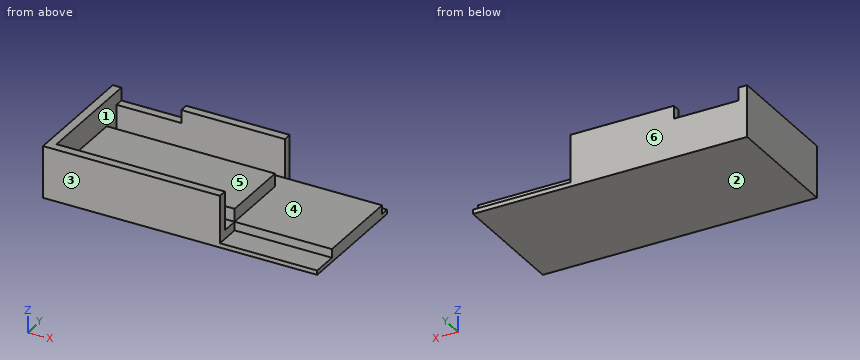
```python
from build123d import *

# Parameters (mm, degrees)
F0_W     = 39
F0_H     = 4
F0_W_2   = 2.54
F0_H_2   = 20.5
F1_DEPTH = 3
F0_H_3   = 16.5
F2_DEPTH = 6
F0_W_3   = 15
F0_H_4   = 2
F3_DEPTH = 9
F0_W_4   = 24
F4_DEPTH = 12
F5_DEPTH = 1


with BuildPart() as f1:
    # F0 (on Top) → F1 (new body)
    with BuildSketch(Plane.XY):
        Polygon((61, 26.5), (41, 26.5), (41, 22.5), (41, 6), (61, 6), align=None)
        Polygon((17, 26.5), (2, 26.5), (2, 22.5), (41, 22.5), (41, 26.5), align=None)
        with Locations((21.5, 4)):
            Rectangle(F0_W, F0_H)
        with Locations((62.27, 16.25)):
            Rectangle(F0_W_2, F0_H_2)
    extrude(amount=F1_DEPTH)

    # F0 (on Top) → F3 (join)
    with BuildSketch(Plane.XY):
        with Locations((9.5, 27.5)):
            Rectangle(F0_W_3, F0_H_4)
    extrude(amount=F3_DEPTH)



with BuildPart() as f2:
    # F0 (on Top) → F2 (new body)
    with BuildSketch(Plane.XY):
        with Locations((21.5, 14.25)):
            Rectangle(F0_W, F0_H_3)
    extrude(amount=F2_DEPTH)


with BuildPart() as f4:
    # F0 (on Top) → F4 (new body)
    with BuildSketch(Plane.XY):
        with Locations((29, 27.5)):
            Rectangle(F0_W_4, F0_H_4)
        Polygon((2, 22.5), (2, 26.5), (2, 28.5), (0, 28.5), (0, 2), (2, 2), (2, 6), align=None)
        Polygon((41, 2), (2, 2), (0, 2), (0, 0), (41, 0), align=None)
    extrude(amount=F4_DEPTH)


with BuildPart() as f1_1:
    add(f1.part)

    add(f2.part)  # F5 merges F2

    add(f4.part)  # F5 merges F4
    # F0 (on Top) → F5 (join)
    with BuildSketch(Plane.XY):
        Polygon((41, 28.5), (41, 26.5), (61, 26.5), (63.54, 26.5), (63.54, 28.5), align=None)
        Polygon((61, 6), (41, 6), (41, 2), (41, 0), (63.54, 0), (63.54, 6), align=None)
    extrude(amount=F5_DEPTH)


solid = f1_1.part
```
Could you check a few things on this model? Use its own coordinates, in mm. Face numbers are marked on the shaded views. A direction names the side the tool comes from. Round coordinates to 2 decimals unless told otherwise and drop trailing zeros. Order: outer loops, then holes, each group sorted by start corner. A loop starts at its lowest first (then second) coordinate and runs counter-clockwise, first axis right, second up. Notation, with made-up numbers: (-1.5, 87.25) -> (32.5, 87.25) arc R30 cw to (32.5, 111.25) -> close; hole circle Ø1 at (12, -9.75). An arc over 180 degrees is marked (long way). One line per question, with ' | ' between items.
Q1. If we section it at A-A on z = 10.25: Write out the boundary of the cut face in (x, y).
Computed values:
outline: (0, 0) -> (41, 0) -> (41, 2) -> (2, 2) -> (2, 28.5) -> (0, 28.5) -> close; (17, 26.5) -> (41, 26.5) -> (41, 28.5) -> (17, 28.5) -> close
Q2. If we section it at B-B on x = 47: Write out the boundary of the cut face in (y, z), plus the area to 3 significant figures.
Computed values:
outline: (0, 0) -> (28.5, 0) -> (28.5, 1) -> (26.5, 1) -> (26.5, 3) -> (6, 3) -> (6, 1) -> (0, 1) -> close | area: 69.5 mm²
Q3. If we section it at D-D on z = 4.75: Write out the boundary of the cut face in (x, y), plus the area to 4 significant figures.
Computed values:
outline: (0, 0) -> (41, 0) -> (41, 2) -> (2, 2) -> (2, 6) -> (41, 6) -> (41, 22.5) -> (2, 22.5) -> (2, 26.5) -> (41, 26.5) -> (41, 28.5) -> (0, 28.5) -> close | area: 856.5 mm²
Q4. If we section it at C-C on y = 19: Write out the boundary of the cut face in (x, z), plus the area to 3 significant figures.
Computed values:
outline: (0, 0) -> (63.54, 0) -> (63.54, 3) -> (41, 3) -> (41, 6) -> (2, 6) -> (2, 12) -> (0, 12) -> close | area: 326 mm²
Q5. Which directions (+Z, -Z, +X, -X, +Y, -Y) give clear straight access to the entire face, cutting with the end or side of a thin tool? Please do the marked faces 5 and 6.
Computed values:
face 5: +Z, +X | face 6: +Z, -Z, +X, -X, +Y
Q6. I'm going to push flat-ended pins straight in: pin 1 (1.2 mm diameter, centred on x = 24, y = 4.5, fed in from +Z); pin 2 (8 mm diameter, centred on x = 22.5, y = 14.5, fed in from +Z); pin 3 (0.6 mm diameter, centred on x = 57, z = 1.5, fed in from +Y). Where does each tip first touch, or does it pass through?
Computed values:
pin 1: z = 3 | pin 2: z = 6 | pin 3: y = 26.5
Q7. If I drill on line 1 (Y direction, x = 17, z = 4.5); line 2 (Y direction, x = 5, z = 9.25), over which ranges is the centre line in solid material (lowest first)? Write a range as from..to.
Computed values:
line 1: 0..2, 6..22.5, 26.5..28.5 | line 2: 0..2
Q8. We'd pull the mould along Y, two halves only. Please class the marked faces 1, 2, 3 and 4: released by +Y, released by -Y, zero draft, split by the parting line, or undercut.
Computed values:
face 1: undercut | face 2: zero draft | face 3: released by -Y | face 4: undercut
